from build123d import *

# Parameters (mm, degrees)
F1_DEPTH = 117.475
F3_D     = 20.6375


# Not quite as in the source:
# - a length typed as a fraction of an inch, garbled in the dataset ("3 / 203.2 mm" for 3/8 in), is restored


with BuildPart() as f1:
    # F0 (on Right) → F1 (new body)
    with BuildSketch(Plane.YZ):
        Polygon((-51.1705551147, 49.2858837724), (-51.1705551147, 182.6358837724), (-68.6330551147, 182.6358837724), (-68.6330551147, 117.5483837724), (-68.6330551147, 49.2858837724), align=None)
        Polygon((-99.7797900677, 49.2858837724), (-68.6330551147, 49.2858837724), (-68.6330551147, 117.5483837724), (-99.7797900677, 117.5483837724), (-99.7797900677, 104.8483837724), (-82.3172900677, 104.8483837724), (-82.3172900677, 61.9858837724), (-99.7797900677, 61.9858837724), align=None)
    extrude(amount=F1_DEPTH)

    # F3 (through all)
    with Locations(Plane(origin=(0, 0, 0), x_dir=(1, 0, 0), z_dir=(0, 1, 0))):
        with Locations((31.75, -150.8858837724), (85.725, -150.8858837724)):
            Hole(F3_D / 2)


solid = f1.part
Can you work these out from the model? Positions are in its coordinate system, mm. A direction names the side the tool comes from. Coordinates: 2 decimals unless noted, no trailing zeros. Write each loop counter-clockwise with the first axis right and the second up, starting at its lowest first coordinate (ties: lowest second). Pieces come first, ordered by that corner, then holes. Notation, with made-up numbers: (-3, -39.75) - (43, -39.75) arc R19 ccw to (43, -17.75) - close; hole circle Ø9 at (23, -37). An arc over 180 degrees is marked (long way). Return JSON: item names as keys, results as strings. Group by question number.
Item 1: Please list where these lines run through material, in increasing order: probe 1 along Z at (x, y) = (31.75, -56.5); probe 2 along Z at (x, y) = (45, -98); probe 3 along Y at (x, z) = (49, 119).
Item 2: Which directions (+Z, -Z, +X, -X, +Y, -Y) give clear straight access to the entire face, cutting with the end or side of a thin tool? Please do faces 1 (the face through (58, -82.317, 84)), 2 (the face through (58, -68.633, 151)), 3 (the face through (33.99, -60.02, 160.96)).
Item 3: If we section it at C-C (z = 95): Write out the boundary of the cut face in (x, y) (3 decimals), then the cut area to 3 significant figures.
Item 4: If we section it at A-A (x = 31.75): Write out the boundary of the cut face in (y, z).
Item 5: I'm going to push flat-ended pins straight in: pin 1 Ø8 at (y, z) = (-61, 107.5) entering from -X; pin 2 Ø8.5 at (x, y) = (62, -95) entering from +Z; pin 3 Ø21.5 at (x, z) = (61, 74.5) entering from -Y. Where does each tip first touch, or does it pass through?
Item 6: If we section it at D-D (y = -71.5): Write out the boundary of the cut face in (x, z) (3 decimals).
Item 7: If we section it at B-B (x = 67.5): Write out the boundary of the cut face in (y, z), then the cut area to 3 significant figures.
Item 8: We'd pull the mould along Z, two halves only. Please class faces 4 (the face through (58, -91, 61.986)), 5 (the face through (58, -76, 49.286)), 6 (the face through (58, -84, 117.548)), 7 (the face through (117.475, -70, 102)): pulls with the +Z half, pulls with the -Z half, needs draft (parallel to the pull), parting line crosses it, or undercut.
Return value:
{
 "1": {"probe 1": "z = 49.29 to 140.57, 161.2 to 182.64", "probe 2": "z = 49.29 to 61.99, 104.85 to 117.55", "probe 3": "y = -68.63 to -51.17"},
 "2": {"face 1": "+X, -X, -Y", "face 2": "+Z, +X, -X, -Y", "face 3": "+Y, -Y"},
 "3": {"outline": "(0, -82.317) - (117.475, -82.317) - (117.475, -51.171) - (0, -51.171) - close", "area": "3,660 mm^2"},
 "4": {"outline": "(-99.78, 49.29) - (-51.17, 49.29) - (-51.17, 140.57) - (-68.63, 140.57) - (-68.63, 117.55) - (-99.78, 117.55) - (-99.78, 104.85) - (-82.32, 104.85) - (-82.32, 61.99) - (-99.78, 61.99) - close; (-68.63, 161.2) - (-51.17, 161.2) - (-51.17, 182.64) - (-68.63, 182.64) - close"},
 "5": {"pin 1": "stops at x = 0", "pin 2": "stops at z = 117.55", "pin 3": "stops at y = -82.32"},
 "6": {"outline": "(0, 49.286) - (117.475, 49.286) - (117.475, 117.548) - (0, 117.548) - close"},
 "7": {"outline": "(-99.78, 49.29) - (-51.17, 49.29) - (-51.17, 182.64) - (-68.63, 182.64) - (-68.63, 117.55) - (-99.78, 117.55) - (-99.78, 104.85) - (-82.32, 104.85) - (-82.32, 61.99) - (-99.78, 61.99) - close", "area": "3,710 mm^2"},
 "8": {"face 4": "undercut", "face 5": "pulls with the -Z half", "face 6": "pulls with the +Z half", "face 7": "needs draft"}
}
